Autodesk Inventor part; units mm, degrees
ref_plane "swivel_to_body_XY" through (0, -10, 0) normal (0, 1, 0) x (1, 0, 0)
ref_plane "swivel_to_body_YZ" through (0, -10, 0) normal (1, 0, 0) x (0, 0, -1)
ref_plane "swivel_to_body_ZX" through (0, -10, 0) normal (0, 0, -1) x (0, 1, 0)
sketch "Sketch_1" plane through (0, 0, 0) normal (0, 1, 0) x (-1, 0, 0)
  arc A0 (35, 12) -> (35, -12) centre (103.9638, 0) ccw
  arc A1 (35, 12) -> (26, 21) centre (26, 12) ccw
  line L0 (26, 21) -> (-26, 21)
  arc A2 (-26, 21) -> (-35, 12) centre (-26, 12) ccw
  arc A3 (-35, -12) -> (-35, 12) centre (-103.9638, 0) ccw
  arc A4 (-35, -12) -> (-26, -21) centre (-26, -12) ccw
  line L1 (-26, -21) -> (26, -21)
  arc A5 (26, -21) -> (35, -12) centre (26, -12) ccw
  circle A6 centre (-28, 14) radius 3.25
  circle A7 centre (-28, -14) radius 3.25
  circle A8 centre (28, 14) radius 3.25
  circle A9 centre (28, -14) radius 3.25
extrude "Extrusion1" add sketch "Sketch_1" against normal blind 2
sketch "Sketch2" plane through (0, 0, 0) normal (0, 1, 0) x (1, 0, 0)
  point P0 (0, 0)
hole "Hole1" at (0, 0, 0) direction (0, -1, 0) diameter 33.6 depth 1
sketch "Sketch_4" plane through (0, 0, 0) normal (0, 0, 1) x (1, 0, 0)
  line L0 (0, -10) -> (0, -2)
  line L1 (0, -2) -> (20.5, -2)
  line L2 (20.5, -2) -> (15.8744, -9.0925)
  arc A0 (14.1992, -10) -> (15.8744, -9.0925) centre (14.1992, -8) ccw
  line L3 (14.1992, -10) -> (0, -10)
  line L4 (0, -10) -> (0, -2)
revolve "Revolution1" add sketch "Sketch_4" angle 360 about axis through (0, -10, 0) along (0, -1, 0)
ref_plane "swivel_to_body_XY" through (0, -10, 0) normal (0, 1, 0) x (1, 0, 0)
ref_plane "swivel_to_body_YZ" through (0, -10, 0) normal (1, 0, 0) x (0, 0, -1)
ref_plane "swivel_to_body_ZX" through (0, -10, 0) normal (0, 0, -1) x (0, 1, 0)
properties part number "CHAMJ-E50-Rswivel"
The listing builds one solid part. Answer for the finished solid, in the listing's coordinates (mm). A direction names the side the tool comes from. Coordinates: 2 decimals unless noted, no trailing zeros. Write each loop counter-clockwise with the first axis right and the second up, starting at its lowest first coordinate (ties: lowest second). Pieces come first, ordered by that corner, then holes. Notation, with made-up numbers: M 36,39.5 L 90,39.5 A30 cw 90,63.5 Z; hole C 59,-7.5 d8. An arc over 180 degrees is marked long. Use one line per item in the form item = value.
Item 1: Find the intervals of material crossed by probe 1 along X at (y, z) = (-0.55, 0); probe 2 along Z at (x, y) = (-28, -0.8); probe 3 along X at (y, z) = (-1.75, 14.5), in increasing order.
Model answer:
probe_1 = -33.96 to -16.8, 16.8 to 33.96
probe_2 = -20.77 to -17.25, -10.75 to 10.75, 17.25 to 20.77
probe_3 = -34.65 to -31.21, -24.79 to 24.79, 31.21 to 34.65
Item 2: Find section C-C, the plane x = 28. Give the vertices of the cut face in (y, z), plus the area to 3 significant figures.
Model answer:
outline = M -2,-20.77 L 0,-20.77 L 0,-17.25 L -2,-17.25 Z; M -2,-10.75 L 0,-10.75 L 0,10.75 L -2,10.75 Z; M -2,17.25 L 0,17.25 L 0,20.77 L -2,20.77 Z
area = 57.1 mm2
Item 3: Given P1, Ø7.5, axis at x = 28, z = -14, coming from the +Y side; P2, Ø3, axis at x = 3, z = 0.5, coming from the +Y side; P3, Ø3, axis at x = 7, y = -7, coming from the -Z side; P4, Ø1, axis at x = -24, z = -14.5, coming from the -Y side, each flat-ended and moving along its own axis, determine where each tip first touches the part or whether it passes through.
Model answer:
P1 = 0
P2 = -1
P3 = -16.97
P4 = -2
Item 4: Find section B-B, the plane z = 0. Give the vertices of the cut face in (x, y).
Model answer:
outline = M -33.96,-2 L -20.5,-2 L -15.87,-9.09 A2 ccw -14.2,-10 L 14.2,-10 A2 ccw 15.87,-9.09 L 20.5,-2 L 33.96,-2 L 33.96,0 L 16.8,0 L 16.8,-1 L -16.8,-1 L -16.8,0 L -33.96,0 Z
Item 5: Find section D-D, the plane y = -6.5. Give the vertices of the cut face in (x, z).
Model answer:
outline = C 0,0 d35.13
Item 6: For faces 1 (the face through (-5.046, -0.507, 16.024)), 2 (the face through (0, -10, 0)), determine the directions among +Z, -Z, +X, -X, +Y, -Y from which every point of the face is accessible in a straight line to the end or side of a thin tool.
Model answer:
face_1 = +Y
face_2 = +Z, -Z, +X, -X, -Y
Item 7: Find section A-A, the plane x = 0. Give the vertices of the cut face in (y, z), plus the area to 3 significant figures.
Model answer:
outline = M -10,-14.2 A2 ccw -9.09,-15.87 L -2,-20.5 L -2,-21 L 0,-21 L 0,-16.8 L -1,-16.8 L -1,16.8 L 0,16.8 L 0,21 L -2,21 L -2,20.5 L -9.09,15.87 A2 ccw -10,14.2 Z
area = 336 mm2
Item 8: The mould has two halves that part along Z. Classify faces 3 (the face through (0, -1, -21)), 4 (the face through (-31.1, -0.99, 14.98)), 5 (the face through (32.294, -0.986, 18.434)), 6 (the face through (-33.964, -0.986, 0.169)): released by +Z, released by -Z, zero draft, split by the parting line, or undercut.
Model answer:
face_3 = released by -Z
face_4 = undercut
face_5 = released by +Z
face_6 = undercut
